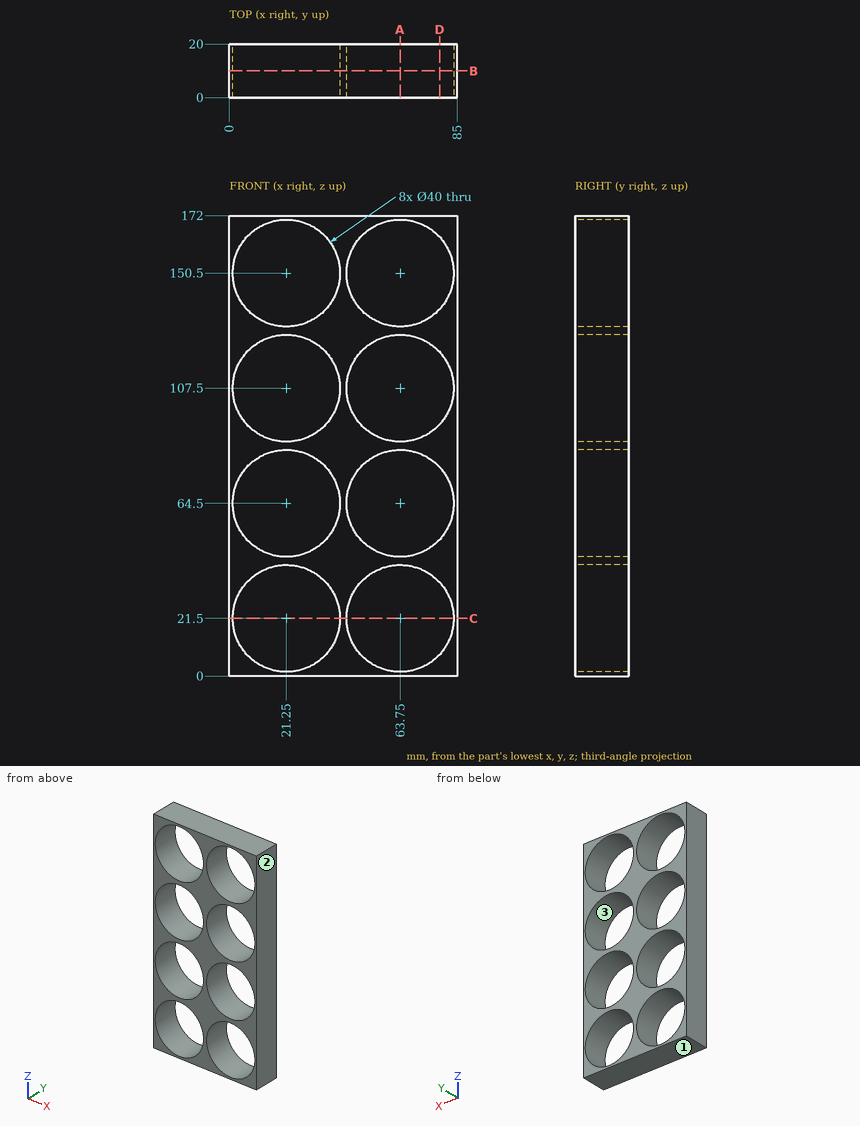
Verification items for this drawing (mm, ordinates from the low corner). Give positions to 0.01 mm unless a question says otherwise; leave off trailing zeros. Order: outer loops, then holes, each group sorted by start corner. A loop starts at its lowest first (then second) coordinate and runs counter-clockwise, first axis right, second up.
1) Material ranges on probe 1 along Z at (x, y) = (21.25, 7.5); probe 2 along X at (y, z) = (5.5, 22); probe 3 along Z at (x, y) = (79.5, 2.25), recorded low to high.
Results are:
probe 1: z = 0 to 1.5, 41.5 to 44.5, 84.5 to 87.5, 127.5 to 130.5, 170.5 to 172
probe 2: x = 0 to 1.26, 41.24 to 43.76, 83.74 to 85
probe 3: z = 0 to 9.17, 33.83 to 52.17, 76.83 to 95.17, 119.83 to 138.17, 162.83 to 172
2) Draft check along Z on the marked faces 1, 2 and 3. Enter one of: released by +Z, released by -Z, zero draft, split by the parting line, or undercut.
Results are:
face 1: released by -Z
face 2: zero draft
face 3: undercut
3) Cross-section at A-A (x = 63.75). Record the boundary of the cut face in (y, z).
Results are:
outline: (0, 0) - (20, 0) - (20, 1.5) - (0, 1.5) - close; (0, 41.5) - (20, 41.5) - (20, 44.5) - (0, 44.5) - close; (0, 84.5) - (20, 84.5) - (20, 87.5) - (0, 87.5) - close; (0, 127.5) - (20, 127.5) - (20, 130.5) - (0, 130.5) - close; (0, 170.5) - (20, 170.5) - (20, 172) - (0, 172) - close
4) Cross-section at D-D (x = 78.5). Record the boundary of the cut face in (y, z).
Results are:
outline: (0, 0) - (20, 0) - (20, 7.99) - (0, 7.99) - close; (0, 35.01) - (20, 35.01) - (20, 50.99) - (0, 50.99) - close; (0, 78.01) - (20, 78.01) - (20, 93.99) - (0, 93.99) - close; (0, 121.01) - (20, 121.01) - (20, 136.99) - (0, 136.99) - close; (0, 164.01) - (20, 164.01) - (20, 172) - (0, 172) - close
5) Cross-section at C-C (z = 21.5). Record the boundary of the cut face in (x, y).
Results are:
outline: (0, 0) - (1.25, 0) - (1.25, 20) - (0, 20) - close; (41.25, 0) - (43.75, 0) - (43.75, 20) - (41.25, 20) - close; (83.75, 0) - (85, 0) - (85, 20) - (83.75, 20) - close
6) Cross-section at B-B (y = 10). Give the number of separate pieces and of enclosed holes in the cut face, then the cut area to 3 significant figures.
Results are:
separate pieces: 1
enclosed holes: 8
area: 4,570 mm2
